Part model, mm, in its own coordinate system. Face numbers are marked on the shaded views. A direction names the side the tool comes from. Coordinates: 2 decimals unless noted, no trailing zeros. Order: outer loops, then holes, each group sorted by start corner. A loop starts at its lowest first (then second) coordinate and runs counter-clockwise, first axis right, second up. Notation, with made-up numbers: M 68,-30 L 103,-30 A15 ccw 103,-24 Z; hole C 10.5,41.25 d8. An arc over 180 degrees is marked long. Answer in a Markdown table with one row per item. Add a question column.
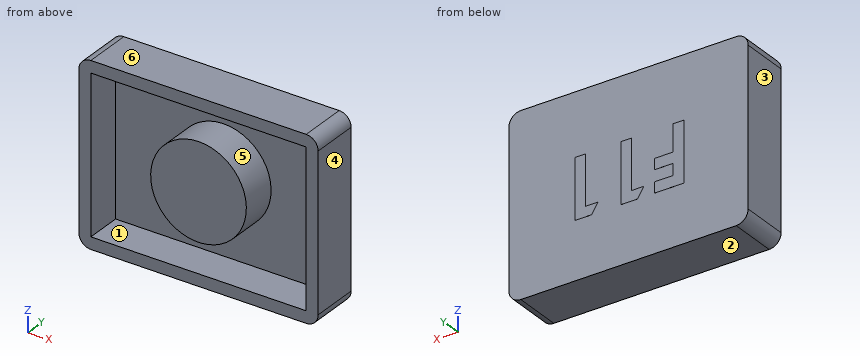
from build123d import *

# Parameters (mm, degrees)
SKETCH1_W           = 12.7
SKETCH1_H           = 9.525
BOSS_EXTRUDE1_DEPTH = 2.54
FILLET1_R           = 0.635
SHELL1_START        = 0.635
SHELL1_OUTLINE_W    = 1.905
SHELL1_OUTLINE_H    = 8.255
SHELL1_DEPTH        = 11.43
SKETCH2_R           = 2.54
BOSS_EXTRUDE2_DEPTH = 1.905
BOSS_EXTRUDE3_DEPTH = 0.00254


# Read off the part's stored shape, not the designer's step: Shell1
with BuildPart() as part:
    # Sketch1 → Boss-Extrude1 (new body)
    with BuildSketch(Plane(origin=(0, 0, 0), x_dir=(1, 0, 0), z_dir=(0, 1, 0))):
        with Locations((6.35, 4.7625)):
            Rectangle(SKETCH1_W, SKETCH1_H)
    extrude(amount=BOSS_EXTRUDE1_DEPTH)

    # Fillet1
    fillet1_edges = [part.edges().sort_by_distance(p)[0] for p in [
        (0, 1.27, -9.525),
        (12.7, 1.27, -9.525),
        (12.7, 1.27, 0),
        (0, 1.27, 0),
    ]]
    fillet(fillet1_edges, radius=FILLET1_R)

    # Shell1 outline → Shell1 (cut)
    with BuildSketch(Plane.YZ.offset(SHELL1_START)):
        with Locations((0.9525, -4.7625)):
            Rectangle(SHELL1_OUTLINE_W, SHELL1_OUTLINE_H)
    extrude(amount=SHELL1_DEPTH, mode=Mode.SUBTRACT)

    # Sketch2 → Boss-Extrude2 (add)
    with BuildSketch(Plane(origin=(0, 1.905, 0), x_dir=(-1, 0, 0), z_dir=(0, -1, 0))):
        with Locations(Location((-6.35, 4.7625, 0), (0, 0, 270))):
            Circle(SKETCH2_R)
    extrude(amount=BOSS_EXTRUDE2_DEPTH)

    # Sketch3 → Boss-Extrude3 (add)
    with BuildSketch(Plane(origin=(0, 2.54, 0), x_dir=(1, 0, 0), z_dir=(0, 1, 0))):
        Polygon((3.414346154, 6.477), (4.961141026, 6.477), (4.961141026, 5.907128205), (3.984217949, 5.907128205), (3.984217949, 5.296551282), (4.961141026, 5.296551282), (4.961141026, 4.726679487), (3.984217949, 4.726679487), (3.984217949, 3.302), (3.414346154, 3.302), align=None)
        Polygon((5.871282252, 6.477), (6.752166667, 6.477), (6.752166667, 3.302), (6.182294872, 3.302), (6.182294872, 5.947833333), (5.531012821, 5.947833333), align=None)
        Polygon((8.313589944, 6.477), (9.194474359, 6.477), (9.194474359, 3.302), (8.624602564, 3.302), (8.624602564, 5.947833333), (7.973320513, 5.947833333), align=None)
    extrude(amount=BOSS_EXTRUDE3_DEPTH)


solid = part.part
(1) Drop a flat-ended pin along its axis: P1, Ø2, axis at x = 2.5, z = -3, coming from the -Y side (3 decimals). Give the stop position or say it passes through.
(2) Slice it at D-D (x = 1). List the corners of the cut face in (y, z) (3 decimals).
(3) 3-axis set-ups, long thin cutter, end or side, ignore diameter. For the marked faces 5 and 6: which of +Z, -Z, +X, -X, +Y, -Y reach the whole face in a straight line?
(4) Pull direction X, two halves, no side cores. Call the marked faces 1, 2, 3 and 4: pulls with the +X half, pulls with the -X half, needs draft (parallel to the pull), parting line crosses it, or undercut.
(5) Slice it at C-C (z = -1.5). List the corners of the cut face in (x, y) (3 decimals).
(6) Wall check: line 1 (Z direction, x = 11.75, y = 0.6) (3 decimals); line 2 (X direction, y = 0.45, z = -5) (3 decimals); line 3 (X direction, y = 1.7, z = -8) (3 decimals). Give the ranges that are in metal, low to high.
(7) Slice it at A-A (y = 1.25). State how many separate pieces and enclosed holes the cut face has, and give its area (3 significant figures).
Computed:
| question | item | result |
|---|---|---|
| 1 | P1 | stops at y = 1.905 |
| 2 | outline | M 0,-9.525 L 2.54,-9.525 L 2.54,0 L 0,0 L 0,-0.635 L 1.905,-0.635 L 1.905,-8.89 L 0,-8.89 Z |
| 3 | face 5 | -Y |
| 3 | face 6 | +Z, +X, -X, +Y, -Y |
| 4 | face 1 | undercut |
| 4 | face 2 | needs draft |
| 4 | face 3 | pulls with the -X half |
| 4 | face 4 | pulls with the +X half |
| 5 | outline | M 0,0 L 0.635,0 L 0.635,1.905 L 12.065,1.905 L 12.065,0 L 12.7,0 L 12.7,2.54 L 0,2.54 Z |
| 6 | line 1 | z = -9.525 to -8.89, -0.635 to 0 |
| 6 | line 2 | x = 0 to 0.635, 3.821 to 8.879, 12.065 to 12.7 |
| 6 | line 3 | x = 0 to 0.635, 12.065 to 12.7 |
| 7 | separate pieces | 2 |
| 7 | enclosed holes | 1 |
| 7 | area | 46.5 mm^2 |
